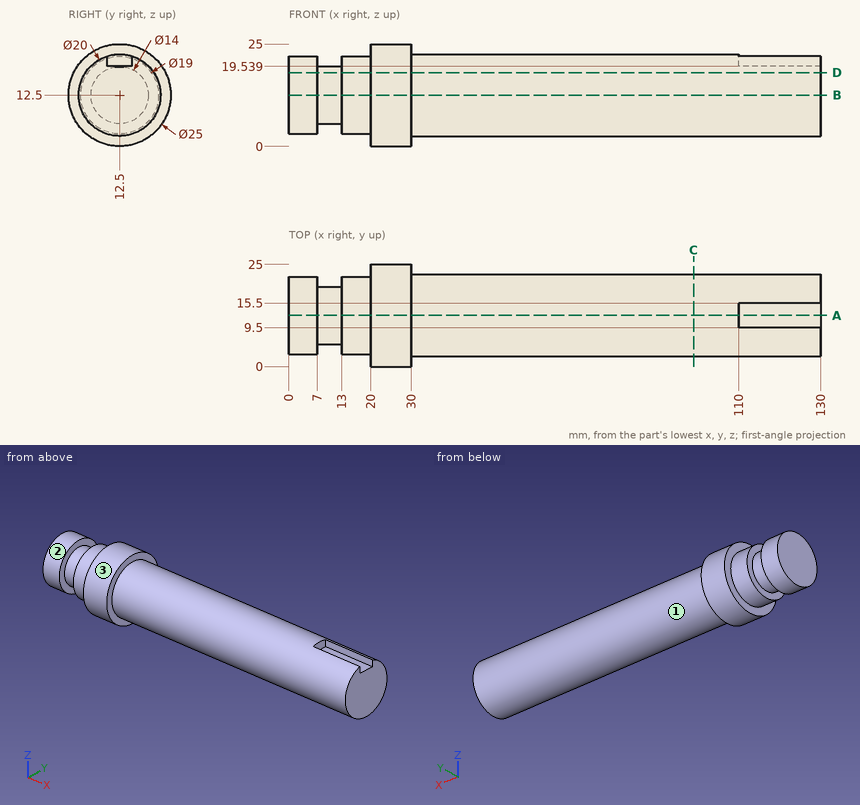
Could you check a few things on this drawing? It's one solid part, dimensions in mm from its lowest x, y, z. A direction names the side the tool comes from. Give positions to 0.01 mm unless a question says otherwise; leave off trailing zeros. Write each loop counter-clockwise with the first axis right and the second up, starting at its lowest first coordinate (ties: lowest second). Pieces come first, ordered by that corner, then holes.
(1) Imagine slicing it at C-C, the plane x = 99. Write out the boundary of the cut face in (y, z).
Output values:
outline: circle Ø20 at (12.5, 12.5)
(2) Imagine slicing it at A-A, the plane y = 12.5. Write out the boundary of the cut face in (x, z), and give its area (3 significant figures).
Output values:
outline: (0, 3) - (7, 3) - (7, 5.5) - (13, 5.5) - (13, 3) - (20, 3) - (20, 0) - (30, 0) - (30, 2.5) - (130, 2.5) - (130, 19.54) - (110, 19.54) - (110, 22.5) - (30, 22.5) - (30, 25) - (20, 25) - (20, 22) - (13, 22) - (13, 19.5) - (7, 19.5) - (7, 22) - (0, 22) - close
area: 2,540 mm2
(3) Imagine slicing it at B-B, the plane z = 12.5. Write out the boundary of the cut face in (x, y).
Output values:
outline: (0, 3) - (7, 3) - (7, 5.5) - (13, 5.5) - (13, 3) - (20, 3) - (20, 0) - (30, 0) - (30, 2.5) - (130, 2.5) - (130, 22.5) - (30, 22.5) - (30, 25) - (20, 25) - (20, 22) - (13, 22) - (13, 19.5) - (7, 19.5) - (7, 22) - (0, 22) - close
(4) On a 3-axis mill with a long thin cutter (end or side, diameter ignored), from which of +Z, -Z, +X, -X, +Y, -Y can I reach the whole of each face in a straight line? I mean the marked faces 1, 2 and 3. Say none if no direction works.
Output values:
face 1: +X
face 2: -X
face 3: +X, -X
(5) If I drill on L1, parallel to X at y = 21, z = 11.25; L2, parallel to Z at x = 34.5, y = 13; L3, parallel to Z at x = 37, y = 19.5, over which ranges is the centre line in solid material (lowest first)?
Output values:
L1: x = 0 to 7, 13 to 130
L2: z = 2.51 to 22.49
L3: z = 5.36 to 19.64
(6) Imagine slicing it at D-D, the plane z = 18. Write out the boundary of the cut face in (x, y) (1 decimal).
Output values:
outline: (0, 4.8) - (7, 4.8) - (7, 8.2) - (13, 8.2) - (13, 4.8) - (20, 4.8) - (20, 1.3) - (30, 1.3) - (30, 4.1) - (130, 4.1) - (130, 20.9) - (30, 20.9) - (30, 23.7) - (20, 23.7) - (20, 20.2) - (13, 20.2) - (13, 16.8) - (7, 16.8) - (7, 20.2) - (0, 20.2) - close
(7) Will these pins go through, and if not, where does the flat tip stop? pin 1 (2 mm diameter, centred on x = 124.5, z = 21, fed in from +Y) (1 decimal); pin 2 (10 mm diameter, centred on x = 79, z = 9.5, fed in from -Y); pin 3 (1.2 mm diameter, centred on x = 124.5, z = 21, fed in from -Y).
Output values:
pin 1: stops at y = 19.1
pin 2: stops at y = 2.5
pin 3: stops at y = 6.37
